Here's how the part is built. I have some questions about the finished solid (model axes, mm). Face numbers are marked on the shaded views. A direction names the side the tool comes from. Coordinates: 2 decimals unless noted, no trailing zeros. Write each loop counter-clockwise with the first axis right and the second up, starting at its lowest first coordinate (ties: lowest second). Pieces come first, ordered by that corner, then holes. Notation, with made-up numbers: (-23, 50) -> (-14, 50) arc R24 cw to (-14, 79) -> close; hole circle Ø4 at (-29.5, 84.5). An arc over 180 degrees is marked (long way). Put each result on its own line as item: value.
```python
from build123d import *

# Parameters (mm, degrees)
SKETCH2_W               = 152.4
SKETCH2_H               = 101.6
BOSS_EXTRUDE1_DEPTH     = 6.35
BOSS_EXTRUDE2_DEPTH     = 8.89
FILLET1_R               = 2.54
SKETCH5_R               = 5.08
CUT_EXTRUDE1_DEPTH      = 192.880455786
MIRROR1_START           = 73.721650485
MIRROR1_OUTLINE_R       = 5.08
MIRROR1_DEPTH           = 8.89
SKETCH12_W              = 44.45
SKETCH12_H              = 27.736089271
BOSS_EXTRUDE4_DEPTH     = 19.05
BOSS_EXTRUDE5_DEPTH     = 8.89
CUT_EXTRUDE4_DEPTH      = 19.05
CUT_EXTRUDE4_DEPTH_BACK = 192.880455786
SKETCH12_4_W            = 19.8882
SKETCH12_4_H            = 14.986
CUT_EXTRUDE5_DEPTH      = 6.35
SKETCH18_W              = 20.32
SKETCH18_H              = 66.04
CUT_EXTRUDE6_DEPTH      = 6.35
SKETCH19_W              = 13.97
SKETCH19_H              = 22.86
CUT_EXTRUDE7_DEPTH      = 184.254753535
SKETCH20_R              = 2.25
SKETCH20_R_2            = 1.1303
CUT_EXTRUDE8_DEPTH      = 184.254753535
SKETCH21_W              = 10.16
SKETCH21_H              = 12.7
BOSS_EXTRUDE6_DEPTH     = 16.51
SKETCH22_W              = 12.7
SKETCH22_H              = 10.16
BOSS_EXTRUDE7_DEPTH     = 22.86
FILLET2_R               = 2.54
FILLET3_R               = 2.54


# Read off the part's stored shape, not the designer's step: Mirror1
with BuildPart() as part:
    # Sketch2 → Boss-Extrude1 (new body)
    with BuildSketch(Plane(origin=(0, 0, 0), x_dir=(1, 0, 0), z_dir=(0, 1, 0))):
        with Locations((42.826537217, -31.811650485)):
            Rectangle(SKETCH2_W, SKETCH2_H)
    extrude(amount=BOSS_EXTRUDE1_DEPTH)

    # Sketch4 → Boss-Extrude2 (add)
    with BuildSketch(Plane(origin=(0, 0, -18.988349515), x_dir=(-1, 0, 0), z_dir=(0, 0, -1))):
        Polygon((-98.179788203, 6.35), (-62.824718494, 85.898906846), (7.885420925, 6.35), (33.373462783, 6.35), (-68.226537217, 120.65), (-119.026537217, 6.35), align=None)
    extrude(amount=-BOSS_EXTRUDE2_DEPTH)

    # Fillet1
    fillet1_edges = [part.edges().sort_by_distance(p)[0] for p in [
        (62.824718494, 85.898906846, -14.543349515),
        (68.226537217, 120.65, -14.543349515),
    ]]
    fillet(fillet1_edges, radius=FILLET1_R)

    # Sketch5 → Cut-Extrude1 (cut, through all)
    with BuildSketch(Plane.XY.offset(-10.098349515)):
        with Locations((61.15629472, 90.616520913)):
            Circle(SKETCH5_R)
    extrude(amount=-CUT_EXTRUDE1_DEPTH, mode=Mode.SUBTRACT)

    # Mirror1 outline → Mirror1 (add)
    with BuildSketch(Plane.XY.offset(MIRROR1_START)):
        with BuildLine():
            ThreePointArc((60.206056328, 82.952911909), (62.494616288, 83.775286431), (64.425557331, 82.297019462))
            Line((64.425557331, 82.297019462), (98.179788203, 6.35))
            Line((98.179788203, 6.35), (119.026537217, 6.35))
            Line((119.026537217, 6.35), (69.827376054, 117.048112617))
            ThreePointArc((69.827376054, 117.048112617), (67.89643501, 118.526379585), (65.607875051, 117.704005063))
            Line((65.607875051, 117.704005063), (-33.373462783, 6.35))
            Line((-33.373462783, 6.35), (-7.885420925, 6.35))
            Line((-7.885420925, 6.35), (60.206056328, 82.952911909))
        make_face()
        with Locations((61.15629472, 90.616520913)):
            Circle(MIRROR1_OUTLINE_R, mode=Mode.SUBTRACT)
    extrude(amount=MIRROR1_DEPTH)

    # Sketch12 → Boss-Extrude4 (add)
    with BuildSketch(Plane(origin=(0, 0, 73.721650485), x_dir=(-1, 0, 0), z_dir=(0, 0, -1))):
        with Locations((11.148462783, 20.218044636)):
            Rectangle(SKETCH12_W, SKETCH12_H)
    extrude(amount=BOSS_EXTRUDE4_DEPTH)

    # Sketch15 → Boss-Extrude5 (add)
    with BuildSketch(Plane.XY.offset(73.721650485)):
        Polygon((-33.373462783, 34.086089271), (-33.373462783, 6.35), (-8.719161209, 34.086089271), align=None)
        Polygon((11.076537217, 27.682202909), (-7.885420925, 6.35), (11.076537217, 6.35), align=None)
    extrude(amount=BOSS_EXTRUDE5_DEPTH)

    # Sketch12<4> → Cut-Extrude4 (cut, two sides: drawn at the far end of the back side and taken through both)
    with BuildSketch(Plane(origin=(0, 0, 73.721650485), x_dir=(-1, 0, 0), z_dir=(0, 0, -1)).offset(-CUT_EXTRUDE4_DEPTH_BACK)):
        with Locations((7.42370528, 13.843)):
            Rectangle(SKETCH12_4_W, SKETCH12_4_H)
    extrude(amount=CUT_EXTRUDE4_DEPTH + CUT_EXTRUDE4_DEPTH_BACK, mode=Mode.SUBTRACT)

    # Sketch17 → Cut-Extrude5 (cut)
    with BuildSketch(Plane(origin=(0, 6.35, 0), x_dir=(1, 0, 0), z_dir=(0, 1, 0))):
        Polygon((-23.508558608, -40.828650485), (-9.633558608, -40.828650485), (-5.633558608, -40.828650485), (8.241441392, -40.828650485), (8.241441392, -39.431650485), (-23.508558608, -39.431650485), align=None)
        Polygon((-5.633558608, -40.828650485), (-9.633558608, -40.828650485), (-23.508558608, -40.828650485), (-23.508558608, -54.671650485), (-17.36780528, -54.671650485), (2.52039472, -54.671650485), (8.241441392, -54.671650485), (8.241441392, -40.828650485), align=None)
    extrude(amount=-CUT_EXTRUDE5_DEPTH, mode=Mode.SUBTRACT)

    # Sketch18 → Cut-Extrude6 (cut)
    with BuildSketch(Plane(origin=(0, 6.35, 0), x_dir=(1, 0, 0), z_dir=(0, 1, 0))):
        with Locations((92.356537217, -30.274439416)):
            Rectangle(SKETCH18_W, SKETCH18_H)
    extrude(amount=-CUT_EXTRUDE6_DEPTH, mode=Mode.SUBTRACT)

    # Sketch19 → Cut-Extrude7 (cut, through all)
    with BuildSketch(Plane(origin=(0, 6.35, 0), x_dir=(1, 0, 0), z_dir=(0, 1, 0))):
        with Locations((-18.768462783, -8.951650485)):
            Rectangle(SKETCH19_W, SKETCH19_H)
    extrude(amount=-CUT_EXTRUDE7_DEPTH, mode=Mode.SUBTRACT)

    # Sketch20 → Cut-Extrude8 (cut, through all)
    # profile 1 of 8: a face of its own
    with BuildSketch(Plane(origin=(0, 6.35, 0), x_dir=(1, 0, 0), z_dir=(0, 1, 0))):
        with Locations(Location((-29.563462783, -6.411650485, 0), (0, 0, 270))):
            Circle(SKETCH20_R)
        with Locations((-29.563462783, -6.411650485)):
            Circle(SKETCH20_R_2, mode=Mode.SUBTRACT)
    # profile 2 of 8: a face of its own
    with BuildSketch(Plane(origin=(0, 6.35, 0), x_dir=(1, 0, 0), z_dir=(0, 1, 0))):
        with Locations((-29.563462783, -6.411650485)):
            Circle(SKETCH20_R_2)
    # profile 3 of 8: a face of its own
    with BuildSketch(Plane(origin=(0, 6.35, 0), x_dir=(1, 0, 0), z_dir=(0, 1, 0))):
        with Locations(Location((-28.293462783, -44.511650485, 0), (0, 0, 270))):
            Circle(SKETCH20_R)
        with Locations((-28.293462783, -44.511650485)):
            Circle(SKETCH20_R_2, mode=Mode.SUBTRACT)
    # profile 4 of 8: a face of its own
    with BuildSketch(Plane(origin=(0, 6.35, 0), x_dir=(1, 0, 0), z_dir=(0, 1, 0))):
        with Locations((-28.293462783, -44.511650485)):
            Circle(SKETCH20_R_2)
    # profile 5 of 8: a face of its own
    with BuildSketch(Plane(origin=(0, 6.35, 0), x_dir=(1, 0, 0), z_dir=(0, 1, 0))):
        with Locations(Location((108.866537217, -0.061650485, 0), (0, 0, 270))):
            Circle(SKETCH20_R)
        with Locations((108.866537217, -0.061650485)):
            Circle(SKETCH20_R_2, mode=Mode.SUBTRACT)
    # profile 6 of 8: a face of its own
    with BuildSketch(Plane(origin=(0, 6.35, 0), x_dir=(1, 0, 0), z_dir=(0, 1, 0))):
        with Locations((108.866537217, -0.061650485)):
            Circle(SKETCH20_R_2)
    # profile 7 of 8: a face of its own
    with BuildSketch(Plane(origin=(0, 6.35, 0), x_dir=(1, 0, 0), z_dir=(0, 1, 0))):
        with Locations(Location((108.866537217, -63.561650485, 0), (0, 0, 270))):
            Circle(SKETCH20_R)
        with Locations((108.866537217, -63.561650485)):
            Circle(SKETCH20_R_2, mode=Mode.SUBTRACT)
    # profile 8 of 8: a face of its own
    with BuildSketch(Plane(origin=(0, 6.35, 0), x_dir=(1, 0, 0), z_dir=(0, 1, 0))):
        with Locations((108.866537217, -63.561650485)):
            Circle(SKETCH20_R_2)
    extrude(amount=-CUT_EXTRUDE8_DEPTH, mode=Mode.SUBTRACT)

    # Sketch21 → Boss-Extrude6 (add)
    with BuildSketch(Plane(origin=(0, 6.35, 0), x_dir=(1, 0, 0), z_dir=(0, 1, 0))):
        with Locations((34.258952171, -26.223650485)):
            Rectangle(SKETCH21_W, SKETCH21_H)
    extrude(amount=BOSS_EXTRUDE6_DEPTH)

    # Sketch22 → Boss-Extrude7 (add)
    with BuildSketch(Plane(origin=(39.338952171, 0, 0), x_dir=(0, 0, -1), z_dir=(1, 0, 0))):
        with Locations((-26.223650485, 17.78)):
            Rectangle(SKETCH22_W, SKETCH22_H)
    extrude(amount=-BOSS_EXTRUDE7_DEPTH)

    # Fillet2
    fillet2_edges = [part.edges().sort_by_distance(p)[0] for p in [
        (39.338952171, 22.86, 26.223650485),
    ]]
    fillet(fillet2_edges, radius=FILLET2_R)

    # Fillet3
    fillet3_edges = [part.edges().sort_by_distance(p)[0] for p in [
        (11.076537217, 20.218044635, 54.671650485),
        (-33.373462783, 20.218044635, 54.671650485),
        (-33.373462783, 3.175, -18.988349515),
        (119.026537217, 3.175, -18.988349515),
        (119.026537217, 3.175, 82.611650485),
        (-33.373462783, 17.043044635, 82.611650485),
    ]]
    fillet(fillet3_edges, radius=FILLET3_R)


solid = part.part
```
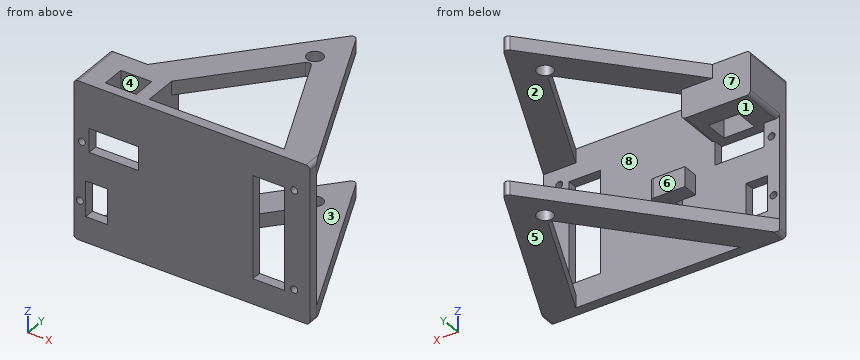
Item 1: Imagine slicing it at A-A on z = 18. Write out the boundary of the cut face in (x, y), then the cut area to 3 significant figures.
Output:
outline: (-33.37, 0) -> (-25.75, 0) -> (-25.75, 6.35) -> (-33.37, 6.35) -> close; (-11.78, 0) -> (82.2, 0) -> (82.2, 6.35) -> (-11.78, 6.35) -> close; (102.52, 0) -> (119.03, 0) -> (119.03, 6.35) -> (102.52, 6.35) -> close
area: 750 mm²
Item 2: Imagine slicing it at D-D on y = 80.5. Write out the boundary of the cut face in (x, z), then the cut area to 3 significant figures.
Output:
outline: (32.54, -18.99) -> (58.03, -18.99) -> (58.03, -10.1) -> (32.54, -10.1) -> close; (32.54, 73.72) -> (58.03, 73.72) -> (58.03, 82.61) -> (32.54, 82.61) -> close; (65.22, -18.99) -> (86.07, -18.99) -> (86.07, -10.1) -> (65.22, -10.1) -> close; (65.22, 73.72) -> (86.07, 73.72) -> (86.07, 82.61) -> (65.22, 82.61) -> close
area: 824 mm²
Item 3: Imagine slicing it at B-B on z = 70. Write out the boundary of the cut face in (x, y), then the cut area to 3 significant figures.
Output:
outline: (-33.37, 0) -> (119.03, 0) -> (119.03, 6.35) -> (11.08, 6.35) -> (11.08, 34.09) -> (-33.37, 34.09) -> close; hole (-17.37, 6.35) -> (2.52, 6.35) -> (2.52, 21.34) -> (-17.37, 21.34) -> close
area: 1,900 mm²
Item 4: Imagine slicing it at C-C on x = 22.5. Write out the boundary of the cut face in (y, z).
Output:
outline: (0, -18.99) -> (6.35, -18.99) -> (6.35, 82.61) -> (0, 82.61) -> close; (12.7, 19.87) -> (22.86, 19.87) -> (22.86, 32.57) -> (12.7, 32.57) -> close; (40.53, -18.99) -> (69.21, -18.99) -> (69.21, -10.1) -> (40.53, -10.1) -> close; (40.53, 73.72) -> (69.21, 73.72) -> (69.21, 82.61) -> (40.53, 82.61) -> close
Item 5: Please list where these lines run through material, in increasing order: line 1 along X through (y, z) = (18.5, 77); line 2 along Z through (x, y) = (44, 93); line 3 along Y through (x, z) = (-8.5, 58.5). Write a range as from..to.
Output:
line 1: x = -33.37..-17.37, 2.52..11.08, 92.78..113.63
line 2: z = -18.99..-10.1, 73.72..82.61
line 3: y = 0..6.35, 21.34..34.09
Item 6: Which directions (+Z, -Z, +X, -X, +Y, -Y) give clear straight access to the entire face, cutting with the end or side of a thin tool? Please do the marked faces 1, 2, 3 and 4.
Output:
face 1: +Y
face 2: +X, +Y
face 3: +X, -X, +Y
face 4: +Z
Item 7: For P1, Ø7, axis at x = 108.87, z = 63.56, coming from the -Y side; P2, Ø5, axis at y = 20, z = 26.5, coming from the -X side; P3, Ø3.5, axis at x = -28.29, z = 44.51, coming from the +Y side; P4, Ø18, axis at x = 32.5, y = 18.5, coming from the -Z side, each with a flat end and sliding along its axis, tell me the tip position at first contact or that it passes through.
Output:
P1: stops at y = 0
P2: stops at x = 16.48
P3: passes through
P4: stops at z = 19.87
Item 8: If we mould it in two halves opening along Z, with no side actions, what happens to the marked faces 5, 6, 7 and 8? For each: released by +Z, released by -Z, zero draft, split by the parting line, or undercut.
Output:
face 5: released by -Z
face 6: zero draft
face 7: undercut
face 8: undercut
